```python
from build123d import *

# Parameters (mm, degrees)
SKETCH1_R           = 31.25
BOSS_EXTRUDE1_DEPTH = 23
SKETCH6_R           = 4
CUT_EXTRUDE3_DEPTH  = 50.820929337
SKETCH7_R           = 4.9
CUT_EXTRUDE4_DEPTH  = 11.5
SKETCH2_R           = 2.125
CUT_EXTRUDE2_DEPTH  = 50.820929337
SKETCH8_R           = 2.85
SKETCH8_R_2         = 2.125
CUT_EXTRUDE5_DEPTH  = 14.5
SKETCH9_R           = 3.625
CUT_EXTRUDE6_DEPTH  = 5
BOSS_EXTRUDE2_START = 4.5
SKETCH10_R          = 31.25
SKETCH10_R_2        = 3.625
SKETCH10_R_3        = 4.9
BOSS_EXTRUDE2_DEPTH = 4.5


with BuildPart() as part:
    # Sketch1 → Boss-Extrude1 (new body)
    with BuildSketch(Plane(origin=(0, 0, 0), x_dir=(0, 0, -1), z_dir=(1, 0, 0))):
        Circle(SKETCH1_R)
    extrude(amount=BOSS_EXTRUDE1_DEPTH)

    # Sketch6 → Cut-Extrude3 (cut, through all)
    with BuildSketch(Plane(origin=(23, 0, 0), x_dir=(0, 0, -1), z_dir=(1, 0, 0))):
        with Locations((-5.435199947, 20.284442352)):
            Circle(SKETCH6_R)
        with Locations((20.284442352, 5.435199947)):
            Circle(SKETCH6_R)
        with Locations((5.435199947, -20.284442352)):
            Circle(SKETCH6_R)
        with Locations((-20.284442352, -5.435199947)):
            Circle(SKETCH6_R)
    extrude(amount=-CUT_EXTRUDE3_DEPTH, mode=Mode.SUBTRACT)

    # Sketch7 → Cut-Extrude4 (cut)
    with BuildSketch(Plane(origin=(23, 0, 0), x_dir=(0, 0, -1), z_dir=(1, 0, 0))):
        with Locations((-5.435199947, 20.284442352)):
            Circle(SKETCH7_R)
        with Locations((20.284442352, 5.435199947)):
            Circle(SKETCH7_R)
        with Locations((5.435199947, -20.284442352)):
            Circle(SKETCH7_R)
        with Locations((-20.284442352, -5.435199947)):
            Circle(SKETCH7_R)
    extrude(amount=-CUT_EXTRUDE4_DEPTH, mode=Mode.SUBTRACT)

    # Sketch2 → Cut-Extrude2 (cut, through all)
    with BuildSketch(Plane(origin=(23, 0, 0), x_dir=(0, 0, -1), z_dir=(1, 0, 0))):
        with Locations((-9.899494937, 9.899494937)):
            Circle(SKETCH2_R)
        with Locations((3.623466631, 13.522961568)):
            Circle(SKETCH2_R)
        with Locations((9.899494937, -9.899494937)):
            Circle(SKETCH2_R)
        with Locations((-3.623466631, -13.522961568)):
            Circle(SKETCH2_R)
    extrude(amount=-CUT_EXTRUDE2_DEPTH, mode=Mode.SUBTRACT)

    # Sketch8 → Cut-Extrude5 (cut)
    # profile 1 of 8: a face of its own
    with BuildSketch(Plane(origin=(23, 0, 0), x_dir=(0, 0, -1), z_dir=(1, 0, 0))):
        with Locations((-9.899494937, 9.899494937)):
            Circle(SKETCH8_R)
        with Locations((-9.899494937, 9.899494937)):
            Circle(SKETCH8_R_2, mode=Mode.SUBTRACT)
    # profile 2 of 8: a face of its own
    with BuildSketch(Plane(origin=(23, 0, 0), x_dir=(0, 0, -1), z_dir=(1, 0, 0))):
        with Locations((-9.899494937, 9.899494937)):
            Circle(SKETCH8_R_2)
    # profile 3 of 8: a face of its own
    with BuildSketch(Plane(origin=(23, 0, 0), x_dir=(0, 0, -1), z_dir=(1, 0, 0))):
        with Locations((3.623466631, 13.522961568)):
            Circle(SKETCH8_R)
        with Locations((3.623466631, 13.522961568)):
            Circle(SKETCH8_R_2, mode=Mode.SUBTRACT)
    # profile 4 of 8: a face of its own
    with BuildSketch(Plane(origin=(23, 0, 0), x_dir=(0, 0, -1), z_dir=(1, 0, 0))):
        with Locations((3.623466631, 13.522961568)):
            Circle(SKETCH8_R_2)
    # profile 5 of 8: a face of its own
    with BuildSketch(Plane(origin=(23, 0, 0), x_dir=(0, 0, -1), z_dir=(1, 0, 0))):
        with Locations((9.899494937, -9.899494937)):
            Circle(SKETCH8_R)
        with Locations((9.899494937, -9.899494937)):
            Circle(SKETCH8_R_2, mode=Mode.SUBTRACT)
    # profile 6 of 8: a face of its own
    with BuildSketch(Plane(origin=(23, 0, 0), x_dir=(0, 0, -1), z_dir=(1, 0, 0))):
        with Locations((9.899494937, -9.899494937)):
            Circle(SKETCH8_R_2)
    # profile 7 of 8: a face of its own
    with BuildSketch(Plane(origin=(23, 0, 0), x_dir=(0, 0, -1), z_dir=(1, 0, 0))):
        with Locations((-3.623466631, -13.522961568)):
            Circle(SKETCH8_R)
        with Locations((-3.623466631, -13.522961568)):
            Circle(SKETCH8_R_2, mode=Mode.SUBTRACT)
    # profile 8 of 8: a face of its own
    with BuildSketch(Plane(origin=(23, 0, 0), x_dir=(0, 0, -1), z_dir=(1, 0, 0))):
        with Locations((-3.623466631, -13.522961568)):
            Circle(SKETCH8_R_2)
    extrude(amount=-CUT_EXTRUDE5_DEPTH, mode=Mode.SUBTRACT)

    # Sketch9 → Cut-Extrude6 (cut)
    with BuildSketch(Plane(origin=(23, 0, 0), x_dir=(0, 0, -1), z_dir=(1, 0, 0))):
        with Locations((-9.899494937, 9.899494937)):
            Circle(SKETCH9_R)
        with Locations((3.623466631, 13.522961568)):
            Circle(SKETCH9_R)
        with Locations((9.899494937, -9.899494937)):
            Circle(SKETCH9_R)
        with Locations((-3.623466631, -13.522961568)):
            Circle(SKETCH9_R)
    extrude(amount=-CUT_EXTRUDE6_DEPTH, mode=Mode.SUBTRACT)

    # Sketch10 → Boss-Extrude2 (add)
    with BuildSketch(Plane(origin=(23, 0, 0), x_dir=(0, 0, -1), z_dir=(1, 0, 0)).offset(BOSS_EXTRUDE2_START)):
        Circle(SKETCH10_R)
        with Locations((-3.623466631, -13.522961568)):
            Circle(SKETCH10_R_2, mode=Mode.SUBTRACT)
        with Locations((-9.899494937, 9.899494937)):
            Circle(SKETCH10_R_2, mode=Mode.SUBTRACT)
        with Locations((-5.435199947, 20.284442352)):
            Circle(SKETCH10_R_3, mode=Mode.SUBTRACT)
        with Locations((20.284442352, 5.435199947)):
            Circle(SKETCH10_R_3, mode=Mode.SUBTRACT)
        with Locations((5.435199947, -20.284442352)):
            Circle(SKETCH10_R_3, mode=Mode.SUBTRACT)
        with Locations((-20.284442352, -5.435199947)):
            Circle(SKETCH10_R_3, mode=Mode.SUBTRACT)
        with Locations((3.623466631, 13.522961568)):
            Circle(SKETCH10_R_2, mode=Mode.SUBTRACT)
        with Locations((9.899494937, -9.899494937)):
            Circle(SKETCH10_R_2, mode=Mode.SUBTRACT)
    extrude(amount=-BOSS_EXTRUDE2_DEPTH)


solid = part.part
```
Can you work these out from the model? Positions are in its coordinate system, mm. A direction names the side the tool comes from. Round coordinates to 2 decimals unless told otherwise and drop trailing zeros. Loops run counter-clockwise (first coordinate to the right, second up) from the corner with the lowest first, then second, coordinate; pieces in that order, holes last.
Item 1: Please list where these lines run through material, in increasing order: L1, parallel to Y at x = 24, z = 8; L2, parallel to Y at x = 25.75, z = 19.5; L3, parallel to Y at x = 14, z = 20.
Item 2: Suppose I cut it at A-A, the plane z = 18. Write out the boundary of the cut face in (x, y), then the cut area to 3 significant figures.
Item 3: Which directions (+Z, -Z, +X, -X, +Y, -Y) give clear straight access to the entire face, cutting with the end or side of a thin tool? Please do faces 1 (the cylindrical face through (4.31, 9.086, 7.937)), 2 (the cylindrical face through (13.317, 15.926, -5.156)).
Item 4: Will these pins go through, and if not, where does the flat tip stop? pin 1 Ø4 at (x, z) = (22, 24) entering from +Y; pin 2 Ø9 at (y, z) = (5.44, -20.28) entering from +X; pin 3 Ø5 at (x, z) = (8.5, -10) entering from +Y.
Item 5: If we mould it in two halves opening along Y, with no side actions, what happens to faces 3 (the flat face through (11.5, -20, -1)), 4 (the flat face through (0, 0, 0))? For each: +Y half, -Y half, draft (parallel to the pull), parting line (faces both ways), or undercut.
Item 6: Suppose I cut it at D-D, the plane x = 3.25. State how many separate pieces and enclosed holes the cut face has, then the cut area to 3 significant figures.
Item 7: Suppose I cut it at C-C, the plane z = 5. Write out the boundary of the cut face in (x, y), then the cut area to 3 significant figures.
Item 8: Suppose I cut it at B-B, the plane y = -23. Write out the boundary of the cut face in (x, z).
Reported:
1. L1: y = -30.21 to 6.81, 12.99 to 16.11, 24.46 to 30.21
1. L2: y = -24.42 to -10.27, -0.6 to 24.42
1. L3: y = -24.01 to -10.33, -0.54 to 24.01
2. outline: (0, -25.55) - (27.5, -25.55) - (27.5, -9.77) - (11.5, -9.77) - (11.5, -8.72) - (0, -8.72) - close; (0, -2.15) - (11.5, -2.15) - (11.5, -1.1) - (27.5, -1.1) - (27.5, 25.55) - (0, 25.55) - close
2. area: 1,190 mm2
3. face 1: +X, -X
3. face 2: +X
4. pin 1: stops at y = 22.19
4. pin 2: stops at x = 11.5
4. pin 3: stops at y = 30.34
5. face 3: undercut
5. face 4: draft
6. separate pieces: 1
6. enclosed holes: 8
6. area: 2,810 mm2
7. outline: (0, -30.85) - (27.5, -30.85) - (27.5, -16.88) - (18, -16.88) - (18, -16.02) - (8.5, -16.02) - (8.5, -15.14) - (0, -15.14) - close; (0, -11.9) - (8.5, -11.9) - (8.5, -11.03) - (18, -11.03) - (18, -10.17) - (27.5, -10.17) - (27.5, 15.4) - (11.5, 15.4) - (11.5, 16.31) - (0, 16.31) - close; (0, 24.26) - (11.5, 24.26) - (11.5, 25.17) - (27.5, 25.17) - (27.5, 30.85) - (0, 30.85) - close
7. area: 1,310 mm2
8. outline: (0, -21.16) - (27.5, -21.16) - (27.5, -9.51) - (11.5, -9.51) - (11.5, -8.37) - (0, -8.37) - close; (0, -2.5) - (11.5, -2.5) - (11.5, -1.36) - (27.5, -1.36) - (27.5, 21.16) - (0, 21.16) - close
